Input: part model. Units: mm. Frame: model coordinates. A direction names the side the tool comes from. Give positions to 0.01 mm unless a question says otherwise; leave off trailing zeros. Loops run counter-clockwise (first coordinate to the right, second up) from the corner with the lowest first, then second, coordinate; pieces in that order, holes last. Notation, with made-up numbers: M 4.5,84 L 47.5,84 A20 ccw 47.5,98 Z; hole C 70.25,83 d10. An arc over 180 degrees is marked long. Answer as a JSON object with one key per item and string values. Group by question number.
1) Draft query along X for faces 1 (the flat face through (20, 4, 0)), 2 (the flat face through (403, -360, 1)), 3 (the flat face through (-405, 4, 397)). Return one class per face: +X half, -X half, draft (parallel to the pull), parting line (faces both ways), or undercut.
2) First-contact query: P1, Ø4, axis at x = 26.5, y = 250, coming from the +Z side; P2, Ø3, axis at y = -213.5, z = 513.5, coming from the -X side; P3, Ø3, axis at y = 188.5, z = 446, coming from the +X side. Flat tips, straight axial feed; report the tip coordinate or a pass-through.
3) Ray query, L1, parallel to Z at x = 321, y = -10; L2, parallel to X at y = 167, z = 263.5; L3, parallel to Z at x = -475.5, y = -208. Return the intervals inside material, ascending.
4) Section query D-D on x = -362. Return loops of the section in (y, z), plus the area to 3 significant figures.
5) Section query A-A on y = -271.5. Return loops of the section in (x, z).
6) Section query B-B on x = -240.5. Return loops of the section in (y, z), plus the area to 3 significant figures.
7) Access query for faces 4 (the flat face through (-7, -300, 233)), 5 (the flat face through (489, 4, 0)), 6 (the flat face through (218, 4, 350)). Directions: +Z, -Z, +X, -X, +Y, -Y. A direction counts if a zero-diameter tool reaches every point of the face in a straight line with its end or side. Return the directions, or none.
8) Section query C-C on z = 301. Return loops of the section in (x, y), plus the area to 3 significant figures.
from build123d import *

# Parameters (mm, degrees)
F0_W     = 1050
F0_H     = 600
F1_DEPTH = 350
F2_W     = 444.603228569
F2_H     = 600
F3_DEPTH = 610
F4_R     = 50
F5_DEPTH = 360
F6_W     = 600
F6_H     = 432.8142261505
F7_DEPTH = 120


with BuildPart() as f1:
    # F0 (on Top) → F1 (new body)
    with BuildSketch(Plane.XY):
        Rectangle(F0_W, F0_H)
    extrude(amount=F1_DEPTH)

    # F2 (on face) → F3 (join)
    with BuildSketch(Plane(origin=(0, 0, 0), x_dir=(1, 0, 0), z_dir=(0, 0, -1))):
        with Locations((-302.6983857155, 0)):
            Rectangle(F2_W, F2_H)
    extrude(amount=-F3_DEPTH)

    # F4 (on Front) → F5 (join, symmetric)
    with BuildSketch(Plane.XZ):
        with Locations((-354.8299782291, 0)):
            Circle(F4_R)
        with Locations((403.5670862999, 0)):
            Circle(F4_R)
    extrude(amount=F5_DEPTH, both=True)

    # F6 (on face) → F7 (cut)
    with BuildSketch(Plane(origin=(-525, 0, 0), x_dir=(0, -1, 0), z_dir=(-1, 0, 0))):
        with Locations((0, 393.5928869247)):
            Rectangle(F6_W, F6_H)
    extrude(amount=-F7_DEPTH, mode=Mode.SUBTRACT)


solid = f1.part
Output:
{
 "1": {"face 1": "undercut", "face 2": "draft", "face 3": "-X half"},
 "2": {"P1": "stops at z = 350", "P2": "stops at x = -405", "P3": "stops at x = -80.4"},
 "3": {"L1": "z = 0 to 350", "L2": "x = -405 to 525", "L3": "z = 0 to 177.19"},
 "4": {"outline": "M -360,-49.48 L 360,-49.48 L 360,49.48 L 300,49.48 L 300,610 L -300,610 L -300,49.48 L -360,49.48 Z", "area": "408,000 mm^2"},
 "5": {"outline": "M -525,0 L -404.83,0 A50 ccw -304.83,0 L 353.57,0 A50 ccw 453.57,0 L 525,0 L 525,350 L -80.4,350 L -80.4,610 L -405,610 L -405,177.19 L -525,177.19 Z"},
 "6": {"outline": "M -300,0 L 300,0 L 300,610 L -300,610 Z", "area": "366,000 mm^2"},
 "7": {"face 4": "+Z, -Y", "face 5": "-Z, +X, +Y, -Y", "face 6": "+Z, +X, +Y, -Y"},
 "8": {"outline": "M -405,-300 L 525,-300 L 525,300 L -405,300 Z", "area": "558,000 mm^2"}
}
